Geometry check sheet. Reference: the model listing, model coordinates, mm. A direction names the side the tool comes from. Coordinates: 2 decimals unless noted, no trailing zeros. Write each loop counter-clockwise with the first axis right and the second up, starting at its lowest first coordinate (ties: lowest second). Pieces come first, ordered by that corner, then holes. Notation, with made-up numbers: M 56.5,56 L 63.5,56 A15 ccw 63.5,74 Z; hole C 60.5,20 d11. An arc over 180 degrees is marked long. Put each result on its own line as item: value. Start each with the question number.
1) Mould release check, pull along Y, two halves, no side actions. Record for faces 3 (the cylindrical face through (-1.5, 0.07, 12.55)), 4 (the flat face through (1.3, -1.4, 16)), 5 (the flat face through (-1.36, -2.39, 7.89)): released by +Y, released by -Y, zero draft, split by the parting line, or undercut.
2) Cross-section at A-A on z = 11.5. Record the cut outline in (x, y).
3) Gauge pin test, flat ends, axial feed: pin 1 (1.5 mm diameter, centred on x = 2, z = 6.5, fed in from +Y); pin 2 (3 mm diameter, centred on x = 2, z = 5, fed in from +Y); pin 3 (1.8 mm diameter, centred on x = 0, y = 0, fed in from +Z). Record the tip position at first contact, or that the pin passes through.
4) Scan lines: line 1 along Z through (x, y) = (-0.3, 2); line 2 along Y through (x, z) = (0, -3.5); line 3 along X through (y, z) = (0.25, -0.5). Record each from-to range of solid material in increasing order.
5) Cross-section at D-D on z = -3. Record the cut outline in (x, y), plus the area to 3 significant figures.
6) Set-up check for faces 1 (the flat face through (1.3, -1.4, 0)), 2 (the conical face through (-0.09, -0.4, 7.91)): record each of +Z, -Z, +X, -X, +Y, -Y from which the full face is reachable in a straight line by a thin tool's end or side.
7) Cross-section at C-C on x = 2.3. Record the cut outline in (y, z).
8) Cross-section at B-B on z = 5.5. Record the cut outline in (x, y), plus the area to 3 significant figures.
from build123d import *

# Parameters (mm, degrees)
PAD_DEPTH       = 16
SKETCH001_R     = 1.5
PAD001_DEPTH    = 6
SKETCH002_R     = 1.5
POCKET_DEPTH    = 8.5
CHAMFER_SIZE    = 1.5
CHAMFER001_SIZE = 0.5


with BuildPart() as part:
    # Sketch → Pad (new body)
    with BuildSketch(Plane.XY):
        Polygon((-2.75, -1.587713), (-2.75, 1.587713), (0, 3.175426), (2.75, 1.587713), (2.75, -1.587713), (0, -3.175426), align=None)
    extrude(amount=PAD_DEPTH)

    # Sketch001 (on Face7 of Pad) → Pad001 (new body)
    with BuildSketch(Plane(origin=(0, 0, 0), x_dir=(1, 0, 0), z_dir=(0, 0, -1))):
        Circle(SKETCH001_R)
    extrude(amount=PAD001_DEPTH)

    # Sketch002 (on Face5 of Pad001) → Pocket (cut)
    with BuildSketch(Plane.XY.offset(16)):
        Circle(SKETCH002_R)
    extrude(amount=-POCKET_DEPTH, mode=Mode.SUBTRACT)

    # Chamfer
    chamfer_edges = [part.edges().sort_by_distance(p)[0] for p in [
        (-1.5, 0, 7.5),
    ]]
    chamfer(chamfer_edges, length=CHAMFER_SIZE)

    # Chamfer001
    chamfer001_edges = [part.edges().sort_by_distance(p)[0] for p in [
        (-1.5, 0, -6),
    ]]
    chamfer(chamfer001_edges, length=CHAMFER001_SIZE)


solid = part.part
Answer key:
1. face 3: undercut
1. face 4: zero draft
1. face 5: released by -Y
2. outline: M -2.75,-1.59 L 0,-3.18 L 2.75,-1.59 L 2.75,1.59 L 0,3.18 L -2.75,1.59 Z; hole C 0,0 d3
3. pin 1: stops at y = 2.45
3. pin 2: stops at y = 2.89
3. pin 3: stops at z = 8.4
4. line 1: z = 0 to 16
4. line 2: y = -1.5 to 1.5
4. line 3: x = -1.48 to 1.48
5. outline: C 0,0 d3
5. area: 7.07 mm²
6. face 1: -Z
6. face 2: +Z
7. outline: M -1.85,0 L 1.85,0 L 1.85,16 L -1.85,16 Z
8. outline: M -2.75,-1.59 L 0,-3.18 L 2.75,-1.59 L 2.75,1.59 L 0,3.18 L -2.75,1.59 Z
8. area: 26.2 mm²
